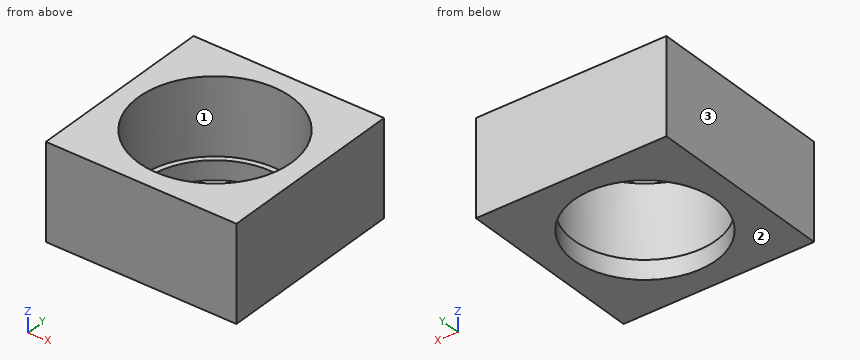
```python
from build123d import *

# Parameters (mm, degrees)
F0_W     = 25.4
F0_H     = 25.4
F1_DEPTH = 12.7
F2_R     = 10.186713
F3_DEPTH = 10.16
F4_R     = 9.458979
F5_DEPTH = 2.54


with BuildPart() as f1:
    # F0 (on Top) → F1 (new body)
    with BuildSketch(Plane.XY):
        with Locations((12.7, -12.7)):
            Rectangle(F0_W, F0_H)
    extrude(amount=F1_DEPTH)

    # F2 (on face) → F3 (cut)
    with BuildSketch(Plane.XY.offset(12.7)):
        with Locations((12.7, -12.7)):
            Circle(F2_R)
    extrude(amount=-F3_DEPTH, mode=Mode.SUBTRACT)

    # F4 (on face) → F5 (cut)
    with BuildSketch(Plane(origin=(0, 0, 0), x_dir=(1, 0, 0), z_dir=(0, 0, -1))):
        with Locations((12.7, 12.7)):
            Circle(F4_R)
    extrude(amount=-F5_DEPTH, mode=Mode.SUBTRACT)


solid = f1.part
```
Verification items for the finished model (mm, model axes). Face numbers are marked on the shaded views. Round coordinates to 2 decimals unless told otherwise and drop trailing zeros. Write each loop counter-clockwise with the first axis right and the second up, starting at its lowest first coordinate (ties: lowest second). Pieces come first, ordered by that corner, then holes. Notation, with made-up numbers: (69.25, 16) -> (73.25, 16) arc R28 cw to (73.25, 44) -> close; hole circle Ø6 at (48.25, 54). An arc over 180 degrees is marked (long way). Write each question's results on one line, items separated by ' | '. Start each with the question number.
1. Cross-section at B-B (x = 12.7). Enter the section's corners in (y, z).
2. Cross-section at C-C (z = 6.75). Enter the section's corners in (x, y).
3. Draft check along X on the marked faces 1, 2 and 3. Enter one of: +X half, -X half, draft (parallel to the pull), parting line (faces both ways), or undercut.
4. Depth check by flat-ended pin: P1, Ø15, axis at x = 12.7, y = -12.7, coming from the -Z side. Enter the tip coordinate at first touch or a pass-through.
5. Material ranges on probe 1 along Y at (x, z) = (12.7, 6.25); probe 2 along X at (y, z) = (-8.25, 9.25); probe 3 along X at (y, z) = (-17.5, 10.5), recorded low to high. Write a range as from..to.
6. Cross-section at A-A (y = -12.7). Enter the section's corners in (x, z), then the cut area to 3 significant figures.
Solutions:
1) outline: (-25.4, 0) -> (-22.16, 0) -> (-22.16, 2.54) -> (-22.89, 2.54) -> (-22.89, 12.7) -> (-25.4, 12.7) -> close; (-3.24, 0) -> (0, 0) -> (0, 12.7) -> (-2.51, 12.7) -> (-2.51, 2.54) -> (-3.24, 2.54) -> close
2) outline: (0, -25.4) -> (25.4, -25.4) -> (25.4, 0) -> (0, 0) -> close; hole circle Ø20.37 at (12.7, -12.7)
3) face 1: undercut | face 2: draft | face 3: -X half
4) P1: passes through
5) probe 1: y = -25.4..-22.89, -2.51..0 | probe 2: x = 0..3.54, 21.86..25.4 | probe 3: x = 0..3.72, 21.68..25.4
6) outline: (0, 0) -> (3.24, 0) -> (3.24, 2.54) -> (2.51, 2.54) -> (2.51, 12.7) -> (0, 12.7) -> close; (22.16, 0) -> (25.4, 0) -> (25.4, 12.7) -> (22.89, 12.7) -> (22.89, 2.54) -> (22.16, 2.54) -> close | area: 67.5 mm2
